Autodesk Inventor part; units mm, degrees
ref_plane "YZ Plane" through (0, 0, 0) normal (1, 0, 0) x (0, 1, 0)
ref_plane "XZ Plane" through (0, 0, 0) normal (0, 1, 0) x (-1, 0, 0)
ref_plane "XY Plane" through (0, 0, 0) normal (0, 0, 1) x (1, 0, 0)
sketch "Boceto1" plane through (0, 0, 0) normal (0, 0, 1) x (1, 0, 0)
  line L0 (20.6547, 17.5) -> (0.4474, -17.5)
  line L1 (-22.6466, -17.5) -> (-2.4393, 17.5)
  circle A0 centre (5.6436, 11.5) radius 2.5
  circle A1 centre (-7.6355, -11.5) radius 2.5
  line L2 (-7, 0) -> (7, 0) construction
  line L3 (-2.4393, 17.5) -> (20.6547, 17.5)
  line L4 (-22.6466, -17.5) -> (0.4474, -17.5)
  point P0 (0, 0)
  point P1 (10.5511, 0)
  point P2 (0, 0)
  dimension "d18" = 60
  dimension "d19" = 10
  dimension "d20" = 10
  dimension "d22" = 20
  dimension "d23" = 6
  dimension "d24" = 6
  dimension "d25" = 2.4393
  dimension "d26" = 5
  dimension "d27" = 14
  dimension "d28" = 35
extrude "Cuerpo lamina" add sketch "Boceto1" along normal blind 2
fillet "R7" radius 7 4 edges at (20.6547, 17.5, 1) (-2.4393, 17.5, 1) (0.4474, -17.5, 1) (-22.6466, -17.5, 1)
sketch "Boceto3" plane through (0, 0, 0) normal (0, 0, -1) x (-1, 0, 0)
  circle A0 centre (-5.6436, 11.5) radius 2.5
  circle A1 centre (7.6355, -11.5) radius 2.5
  point P0 (0, 0)
hole "BCA M5 Izq" at (-7.6355, -11.5, 0) direction (0, 0, 1) diameter 4.134 depth 14.2 tip angle 118 countersink diameter 10 countersink angle 90
sketch "Sketch4" plane through (0, 0, 2) normal (0, 0, 1) x (1, 0, 0)
  circle A0 centre (5.6436, 11.5) radius 2.5
  circle A1 centre (-7.6355, -11.5) radius 2.5
  point P0 (0, 0)
hole "BCA M5 Der" at (5.6436, 11.5, 2) direction (0, 0, -1) diameter 5 depth 14.2 tip angle 118 countersink diameter 10 countersink angle 90
equation "\"d19\" = 0.5 * d22"
equation "\"d20\" = d19"
equation "\"d24\" = d23"
properties part number "Lamina"
The model under review builds one solid part; all positions refer to its coordinate system, in mm. Give positions to 0.01 mm unless a question says otherwise; leave off trailing zeros. Order: outer loops, then holes, each group sorted by start corner. A loop starts at its lowest first (then second) coordinate and runs counter-clockwise, first axis right, second up. Notation, with made-up numbers: M 61.5,55.5 L 109.5,55.5 A13 ccw 109.5,67.5 Z; hole C 34,-19.75 d6. An arc over 180 degrees is marked long. Answer in a Markdown table with one row per item. Add a question column.
1. Add section A-A on y = -11.5. State the section outline as (x, z) points, plus the area to 3 significant figures.
2. Add section B-B on z = 1.2. State the section outline as (x, y) points.
3. To check wall thickness, follow line 1 along X through (y, z) = (10, 1.15); line 2 along Y through (x, z) = (8, 0.9); line 3 along Y through (x, z) = (-11.5, 0.6). State the ranges of each line that lie inside material, in increasing order.
4. Add section D-D on y = -2. State the section outline as (x, z) points, plus the area to 3 significant figures.
5. Add section C-C on x = -15. State the section outline as (y, z) points.
The answers:
| question | item | result |
|---|---|---|
| 1 | outline | M -17.45,0 L -12.64,0 L -10.64,2 L -17.45,2 Z; M -4.64,2 L -2.64,0 L 3.91,0 L 3.91,2 Z |
| 1 | area | 26.7 mm2 |
| 2 | outline | M -16.58,-7 A7 ccw -10.52,-17.5 L -3.59,-17.5 A7 ccw 2.47,-14 L 14.59,7 A7 ccw 8.53,17.5 L 1.6,17.5 A7 ccw -4.46,14 Z; hole C -7.64,-11.5 d7.6; hole C 5.64,11.5 d8.4 |
| 3 | line 1 | -6.77 to 1.77, 9.51 to 15.51 |
| 3 | line 2 | -4.42 to 8.39, 14.61 to 17.5 |
| 3 | line 3 | -17.43 to -13.6, -9.4 to 1.81 |
| 4 | outline | M -13.7,0 L 9.4,0 L 9.4,2 L -13.7,2 Z |
| 4 | area | 46.2 mm2 |
| 5 | outline | M -15.88,0 L -4.26,0 L -4.26,2 L -15.88,2 Z |
